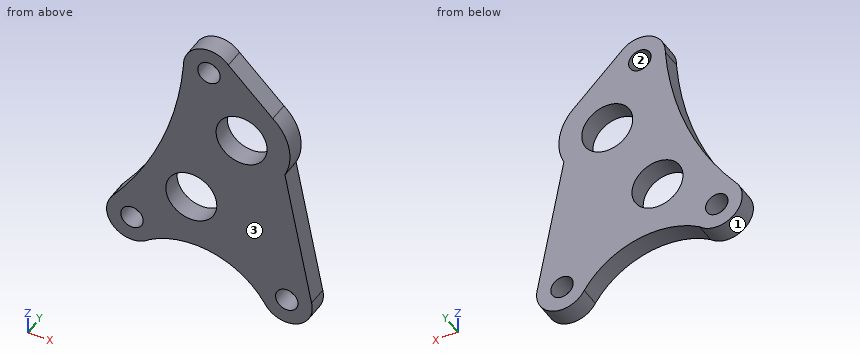
from build123d import *

# Parameters (mm, degrees)
F0_R     = 4.4
F0_R_2   = 10
F1_DEPTH = 8


# Not quite as in the source:
# - a feature names something its author has since deleted; it is built from what else it names


with BuildPart() as f1:
    # F0 (on Front) → F1 (new body)
    with BuildSketch(Plane.XZ):
        with BuildLine():
            Line((31.9492522213, 47.021704051), (14.5416913837, 63.871923339))
            ThreePointArc((14.5416913837, 63.871923339), (3.3211707837, 66.7258087658), (-3.0733272697, 57.0741177632))
            ThreePointArc((-3.0733272697, 57.0741177632), (-11.6409365793, 20.6574209247), (-30.8284920773, -11.4582676391))
            ThreePointArc((-30.8284920773, -11.4582676391), (-30.197435382, -25.1853746986), (-16.4565083148, -25.3218448705))
            ThreePointArc((-16.4565083148, -25.3218448705), (8.288194067, -21.4806704364), (28.7486613668, -35.9175743588))
            ThreePointArc((28.7486613668, -35.9175743588), (41.111240011, -40.2846954641), (47.1716852414, -28.6581697108))
            Line((47.1716852414, -28.6581697108), (36.7147233028, 24.0100747195))
            ThreePointArc((36.7147233028, 24.0100747195), (38.3163132105, 36.3410020894), (31.9492522213, 47.021704051))
        make_face()
        with Locations((-23.2548138211, -17.9881526052)):
            Circle(F0_R, mode=Mode.SUBTRACT)
        Circle(F0_R_2, mode=Mode.SUBTRACT)
        with Locations((37.4451861789, -30.9809301349)):
            Circle(F0_R, mode=Mode.SUBTRACT)
        with Locations((6.9214779515, 57.3964042673)):
            Circle(F0_R, mode=Mode.SUBTRACT)
        with Locations((19.7110784827, 32.4880498807)):
            Circle(F0_R_2, mode=Mode.SUBTRACT)
    extrude(amount=F1_DEPTH)


solid = f1.part
Build history of the part. All positions in model axes, mm. Face numbers are marked on the shaded views. Coordinates: 2 decimals unless noted, no trailing zeros. Write each loop counter-clockwise with the first axis right and the second up, starting at its lowest first coordinate (ties: lowest second). Pieces come first, ordered by that corner, then holes.
(1) Pin check, flat tips, straight feed: pin 1 Ø1 at (x, y) = (-24.5, -3) entering from +Z; pin 2 Ø1 at (y, z) = (-7, 38.5) entering from -X. Stop position of each tip, or through.
(2) Mould opens along Z. For the marked faces 1, 2 and 3 say: pulls with the +Z half, pulls with the -Z half, needs draft (parallel to the pull), parting line crosses it, or undercut.
(3) Cut at A-A on z = 0. List the corners of the cut face in (x, y).
(4) Drill centre lines: line 1 (Z direction, x = 4, y = -5.25); line 2 (X direction, y = -2.75, z = -2.5); line 3 (X direction, y = -1.25, z = 37.5). Where is each one in solid material? Low to high.
(5) Cut at B-B on x = 0. List the corners of the cut face in (y, z), and give its area (3 significant figures).
(6) Cut at D-D on z = 17.5. List the corners of the cut face in (x, y).
(7) Cut at C-C on y = -3. List the corners of the cut face in (x, z).
Working result:
1. pin 1: stops at z = -2.4
1. pin 2: stops at x = -6.08
2. face 1: parting line crosses it
2. face 2: undercut
2. face 3: needs draft
3. outline: (-22.4, -8) - (-10, -8) - (-10, 0) - (-22.4, 0) - close; (10, -8) - (41.48, -8) - (41.48, 0) - (10, 0) - close
4. line 1: z = -20.77 to -9.17, 9.17 to 54.11, 60.69 to 66.96
4. line 2: x = -24.07 to -9.68, 9.68 to 41.98
4. line 3: x = -6.2 to 11.06, 28.36 to 38.04
5. outline: (-8, -20.61) - (0, -20.61) - (0, -10) - (-8, -10) - close; (-8, 10) - (0, 10) - (0, 64.61) - (-8, 64.61) - close
5. area: 522 mm2
6. outline: (-12.97, -8) - (38.01, -8) - (38.01, 0) - (-12.97, 0) - close
7. outline: (-30.83, -11.46) arc R10 ccw to (-16.46, -25.32) arc R33.4 cw to (28.75, -35.92) arc R10 ccw to (47.17, -28.66) - (36.71, 24.01) arc R19 ccw to (31.95, 47.02) - (14.54, 63.87) arc R10 ccw to (-3.07, 57.07) arc R122.15 cw to start; hole circle Ø8.8 at (-23.25, -17.99); hole circle Ø20 at (0, 0); hole circle Ø8.8 at (6.92, 57.4); hole circle Ø20 at (19.71, 32.49); hole circle Ø8.8 at (37.45, -30.98)
